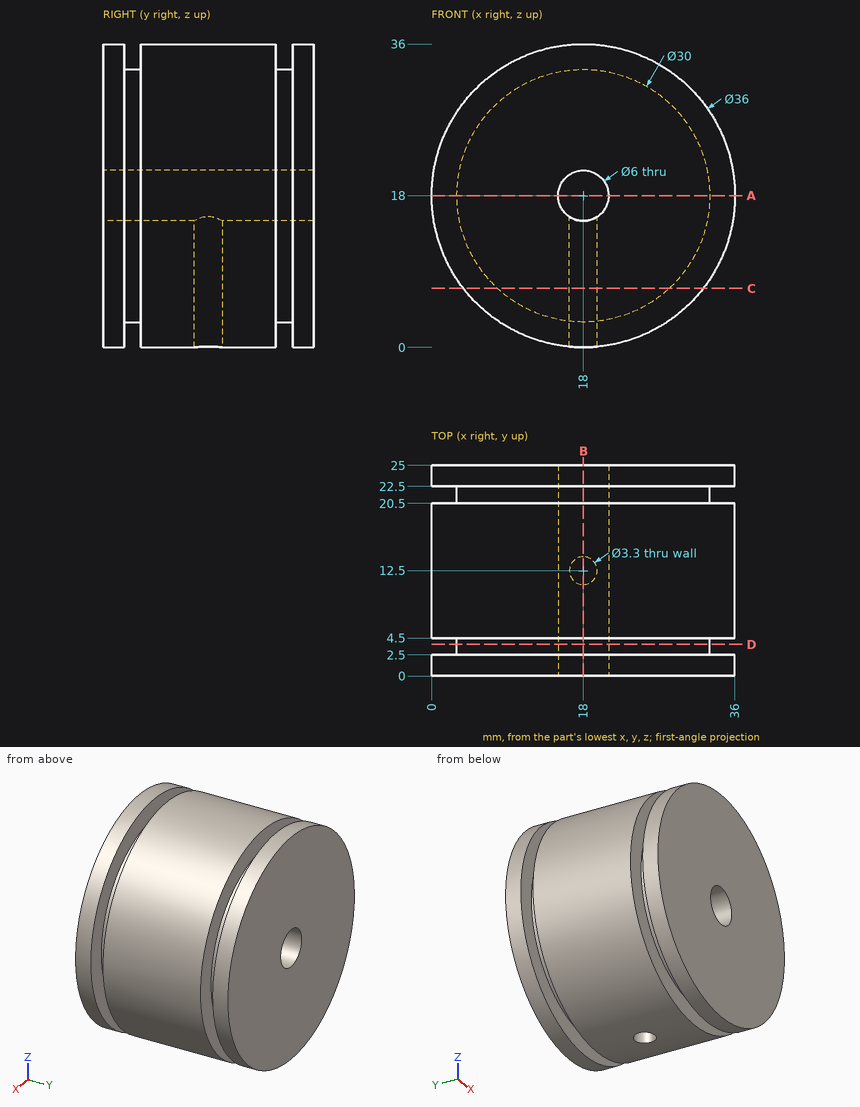
Print and shaded views of the part. All mm, measured from the part's lowest x, y and z. Coordinates: 2 decimals unless noted, no trailing zeros. Loops run counter-clockwise (first coordinate to the right, second up) from the corner with the lowest first, then second, coordinate; pieces in that order, holes last. Notation, with made-up numbers: (56.5, 19) - (108.5, 19) arc R4 ccw to (108.5, 23) - close; hole circle Ø8 at (65, -16.5). An arc over 180 degrees is marked (long way). Use one line per item in the form item = value. Start each with the question number.
1) Band-saw the part on B-B (x = 18). Give the cut face in (y, z).
2) Band-saw the part on C-C (z = 7). Give the cut face in (x, y), and give its area (3 significant figures).
3) Drill centre lines: L1, parallel to Y at x = 8, z = 32; L2, parallel to X at y = 19.75, z = 18; L3, parallel to Z at x = 18.5, y = 7. Where is each one in solid material? Low to high. Write a range as from..to.
4) Flat gauge pins, fed straight in: pin 1 (8 mm diameter, centred on y = 21, z = 19.5, fed in from +X); pin 2 (2 mm diameter, centred on y = 21, z = 19.5, fed in from -X); pin 3 (1.5 mm diameter, centred on x = 20, y = 10.5, fed in from -Z). Where does each tip first touch, or does it go through?
5) Band-saw the part on D-D (y = 3.75). Give the cut face in (x, z), and give its area (3 significant figures).
6) Band-saw the part on A-A (z = 18). Give the cut face in (x, y), and give its area (3 significant figures).
Check values:
q1.outline = (0, 0) - (2.5, 0) - (2.5, 3) - (4.5, 3) - (4.5, 0) - (10.85, 0) - (10.85, 15) - (0, 15) - close; (0, 21) - (25, 21) - (25, 36) - (22.5, 36) - (22.5, 33) - (20.5, 33) - (20.5, 36) - (4.5, 36) - (4.5, 33) - (2.5, 33) - (2.5, 36) - (0, 36) - close; (14.15, 0) - (20.5, 0) - (20.5, 3) - (22.5, 3) - (22.5, 0) - (25, 0) - (25, 15) - (14.15, 15) - close
q2.outline = (3.75, 0) - (32.25, 0) - (32.25, 2.5) - (28.2, 2.5) - (28.2, 4.5) - (32.25, 4.5) - (32.25, 20.5) - (28.2, 20.5) - (28.2, 22.5) - (32.25, 22.5) - (32.25, 25) - (3.75, 25) - (3.75, 22.5) - (7.8, 22.5) - (7.8, 20.5) - (3.75, 20.5) - (3.75, 4.5) - (7.8, 4.5) - (7.8, 2.5) - (3.75, 2.5) - close; hole circle Ø3.3 at (18, 12.5)
q2.area = 671 mm2
q3.L1 = 0..2.5, 4.5..20.5, 22.5..25
q3.L2 = 0..15, 21..36
q3.L3 = 0.01..15.04, 20.96..35.99
q4.pin_1 = 36
q4.pin_2 = 0.01
q4.pin_3 = 0.04
q5.outline = circle Ø30 at (18, 18); hole circle Ø6 at (18, 18)
q5.area = 679 mm2
q6.outline = (0, 0) - (15, 0) - (15, 25) - (0, 25) - (0, 22.5) - (3, 22.5) - (3, 20.5) - (0, 20.5) - (0, 4.5) - (3, 4.5) - (3, 2.5) - (0, 2.5) - close; (21, 0) - (36, 0) - (36, 2.5) - (33, 2.5) - (33, 4.5) - (36, 4.5) - (36, 20.5) - (33, 20.5) - (33, 22.5) - (36, 22.5) - (36, 25) - (21, 25) - close
q6.area = 726 mm2
